The listing builds one solid part. Answer for the finished solid, in the listing's coordinates (mm). A direction names the side the tool comes from. Give positions to 0.01 mm unless a question says otherwise; leave off trailing zeros. Order: outer loops, then holes, each group sorted by start corner. A loop starts at its lowest first (then second) coordinate and runs counter-clockwise, first axis right, second up. Notation, with made-up numbers: (16, -34) - (70, -34) arc R26 cw to (70, -10) - close; hole circle Ø7 at (57, -14). An arc over 180 degrees is marked (long way). Use CSV: the item, a comma, the result in double quotes.
```python
from build123d import *

# Parameters (mm, degrees)
F0_W        = 482.6
F0_H        = 88.9
F0_R        = 5.5372
F1_DEPTH    = 2.54
F2_W        = 450.85
F2_H        = 88.9
F3_DEPTH    = 398.78
F4_DEPTH    = 398.781
F6_D        = 4.0386
F7_T        = 2.54
F7_T3_DEPTH = 93.98


# Not quite as in the source:
# - a shell that OpenCascade refuses in one call is made with other operations: the cavity is built on its own and cut out


with BuildPart() as f1:
    # F0 (on Front) → F1 (new body)
    with BuildSketch(Plane.XZ):
        Rectangle(F0_W, F0_H)
        with Locations((-212.725, -19.05)):
            Circle(F0_R, mode=Mode.SUBTRACT)
        with Locations((-187.325, -19.05)):
            Circle(F0_R, mode=Mode.SUBTRACT)
        with Locations((-155.575, -19.05)):
            Circle(F0_R, mode=Mode.SUBTRACT)
        with Locations((-130.175, -19.05)):
            Circle(F0_R, mode=Mode.SUBTRACT)
        with Locations((-98.425, -19.05)):
            Circle(F0_R, mode=Mode.SUBTRACT)
        with Locations((-73.025, -19.05)):
            Circle(F0_R, mode=Mode.SUBTRACT)
        with Locations((-41.275, -19.05)):
            Circle(F0_R, mode=Mode.SUBTRACT)
        with Locations((-15.875, -19.05)):
            Circle(F0_R, mode=Mode.SUBTRACT)
        with Locations((15.875, -19.05)):
            Circle(F0_R, mode=Mode.SUBTRACT)
        with Locations((41.275, -19.05)):
            Circle(F0_R, mode=Mode.SUBTRACT)
        with Locations((73.025, -19.05)):
            Circle(F0_R, mode=Mode.SUBTRACT)
        with Locations((98.425, -19.05)):
            Circle(F0_R, mode=Mode.SUBTRACT)
        with Locations((130.175, -19.05)):
            Circle(F0_R, mode=Mode.SUBTRACT)
        with Locations((155.575, -19.05)):
            Circle(F0_R, mode=Mode.SUBTRACT)
        with Locations((187.325, -19.05)):
            Circle(F0_R, mode=Mode.SUBTRACT)
        with Locations((212.725, -19.05)):
            Circle(F0_R, mode=Mode.SUBTRACT)
        with Locations((-200.025, 19.05)):
            Circle(F0_R, mode=Mode.SUBTRACT)
        with Locations((-142.875, 19.05)):
            Circle(F0_R, mode=Mode.SUBTRACT)
        with Locations((-85.725, 19.05)):
            Circle(F0_R, mode=Mode.SUBTRACT)
        with Locations((-28.575, 19.05)):
            Circle(F0_R, mode=Mode.SUBTRACT)
        with Locations((28.575, 19.05)):
            Circle(F0_R, mode=Mode.SUBTRACT)
        with Locations((85.725, 19.05)):
            Circle(F0_R, mode=Mode.SUBTRACT)
        with Locations((142.875, 19.05)):
            Circle(F0_R, mode=Mode.SUBTRACT)
        with Locations((200.025, 19.05)):
            Circle(F0_R, mode=Mode.SUBTRACT)
    extrude(amount=F1_DEPTH)

    # F2 (on face) → F3 (join)
    with BuildSketch(Plane(origin=(0, 0, 0), x_dir=(-1, 0, 0), z_dir=(0, 1, 0))):
        Rectangle(F2_W, F2_H)
    extrude(amount=F3_DEPTH)

    # F4 (cut, through all): faces of the model
    f4_faces = [f1.faces().sort_by_distance(p)[0] for p in [
        (-200.025, 0, 19.05),
        (-212.725, 0, -19.05),
        (-187.325, 0, -19.05),
        (-142.875, 0, 19.05),
        (-155.575, 0, -19.05),
        (-130.175, 0, -19.05),
        (-85.725, 0, 19.05),
        (-98.425, 0, -19.05),
        (-73.025, 0, -19.05),
        (-41.275, 0, -19.05),
        (-28.575, 0, 19.05),
        (-15.875, 0, -19.05),
        (15.875, 0, -19.05),
        (28.575, 0, 19.05),
        (41.275, 0, -19.05),
        (73.025, 0, -19.05),
        (85.725, 0, 19.05),
        (98.425, 0, -19.05),
        (130.175, 0, -19.05),
        (142.875, 0, 19.05),
        (155.575, 0, -19.05),
        (187.325, 0, -19.05),
        (200.025, 0, 19.05),
        (212.725, 0, -19.05),
    ]]
    extrude(f4_faces, amount=-F4_DEPTH, mode=Mode.SUBTRACT)

    # F6 (through all)
    with Locations(Plane.XZ.offset(2.54)):
        with Locations((233.3625, -38.1), (233.3625, -6.35), (-233.3625, 22.225), (233.3625, -22.225), (-233.3625, 38.1), (-233.3625, 6.35), (-233.3625, -22.225), (-233.3625, -6.35), (-233.3625, -38.1), (233.3625, 38.1), (233.3625, 22.225), (233.3625, 6.35)):
            Hole(F6_D / 2)

    # F7: shell of thickness 2.54, made by hand


with BuildPart() as f7_core1:
    # F7_t2: copy of F1
    add(f1.part)

    # the walls: a layer under each face that stays
    f7_faces = [f7_core1.faces().sort_by_distance(p)[0] for p in [
        (241.3, -1.27, 0),
        (0, -2.54, 0),
        (-241.3, -1.27, 0),
        (-233.3625, 0, 0),
        (-225.425, 199.39, 0),
        (225.425, 199.39, 0),
        (233.3625, 0, 0),
        (0, 198.12, -44.45),
        (-235.3818, -1.27, -38.1),
        (-235.3818, -1.27, -22.225),
        (-235.3818, -1.27, -6.35),
        (231.3432, -1.27, -38.1),
        (231.3432, -1.27, -22.225),
        (231.3432, -1.27, -6.35),
        (-235.3818, -1.27, 6.35),
        (-235.3818, -1.27, 22.225),
        (-235.3818, -1.27, 38.1),
        (231.3432, -1.27, 6.35),
        (231.3432, -1.27, 22.225),
        (231.3432, -1.27, 38.1),
    ]]
    thicken(f7_faces, amount=-F7_T, mode=Mode.SUBTRACT)

    # F7_s4 → F7_t3 (cut)
    with BuildSketch(Plane.XY.offset(-46.99)):
        Polygon((-225.4504, 0.0254), (-225.425, -2.54), (-222.885, -2.54), (-222.885, 0), align=None)
        Polygon((225.4504, 0.0254), (222.885, 0), (222.885, -2.54), (225.425, -2.54), align=None)
    extrude(amount=F7_T3_DEPTH, mode=Mode.SUBTRACT)


with BuildPart() as f1_1:
    add(f1.part)

    # what is left inside the walls is the cavity
    f7_cavity = [f7_core1.part.solids().sort_by_distance(p)[0] for p in [
        (0, 132.926667, 44.4246),
    ]]
    add(f7_cavity, mode=Mode.SUBTRACT)


solid = f1_1.part
```
Item 1: The part is cut by section A-A (x = 130.5). Give the vertices of the cut face in (y, z), and give its area (3 significant figures).
Taken from the geometry:
outline,"(-2.54, -44.45) - (398.78, -44.45) - (398.78, -41.91) - (0, -41.91) - (0, -24.58) - (-2.54, -24.58) - close; (-2.54, -13.52) - (0, -13.52) - (0, 44.45) - (-2.54, 44.45) - close"
area,"1,210 mm^2"
Item 2: Find the intervals of material crossed by line 1 along X through (y, z) = (-1, -38); line 2 along X through (y, z) = (335, 15) (3 decimals); line 3 along Y through (x, z) = (-176, 15), in increasing order.
Taken from the geometry:
line 1,"-241.3 to -235.38, -231.35 to 231.35, 235.38 to 241.3"
line 2,"-225.425 to -222.885, 222.885 to 225.425"
line 3,"-2.54 to 0"
Item 3: Each of these flat-tipped pins is pushed along its axis until it touches: pin 1 (14.5 mm diameter, centred on x = 41.275, z = -19.05, fed in from +Y); pin 2 (14.5 mm diameter, centred on x = -15.875, z = -19.05, fed in from -Y); pin 3 (8 mm diameter, centred on y = 211, z = -27, fed in from +X) (3 decimals); pin 4 (4 mm diameter, centred on x = 50, y = 147, fed in from +Z). Where does it stop, or does it pass through?
Taken from the geometry:
pin 1,"y = 0"
pin 2,"y = -2.54"
pin 3,"x = 225.425"
pin 4,"z = -41.91"
Item 4: The mould has two halves that part along X. Classify faces 1 (the face through (-3, -2.54, 1)), 2 (the face through (-225.425, 197, -1)), 3 (the face through (3, 197, -41.91)): +X half, -X half, draft (parallel to the pull), parting line (faces both ways), or undercut.
Taken from the geometry:
face 1,"draft"
face 2,"-X half"
face 3,"undercut"
Item 5: The part is cut by section B-B (y = 87.5). Give the vertices of the cut face in (x, z) (3 decimals), and give its area (3 significant figures).
Taken from the geometry:
outline,"(-225.425, -44.45) - (225.425, -44.45) - (225.425, 44.45) - (222.885, 44.45) - (222.885, -41.91) - (-222.885, -41.91) - (-222.885, 44.45) - (-225.425, 44.45) - close"
area,"1,580 mm^2"
Item 6: Which of the six approach directions +Z, -Z, +X, -X, +Y, -Y give full straight-line access (tool end or side, diameter ignored) to faces 4 (the face through (-205.557, -1.252, 19.293)), 5 (the face through (-3, 0, 2)), 6 (the face through (233, 0, 1))?
Taken from the geometry:
face 4,"+Y, -Y"
face 5,"+Z, +Y"
face 6,"+Z, -Z, +X, +Y"
